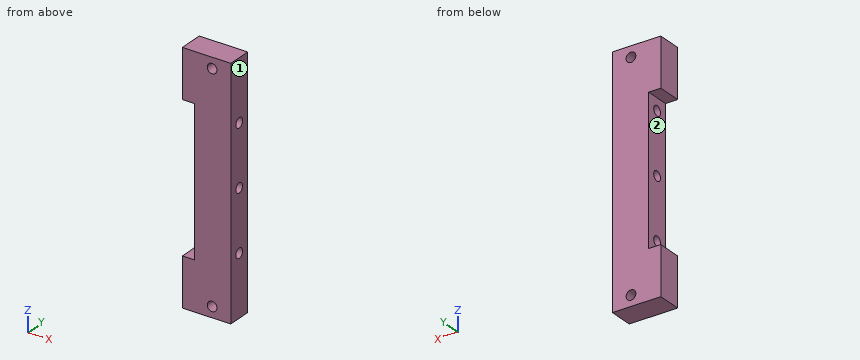
from build123d import *

# Parameters (mm, degrees)
SKETCH1_R           = 2
BOSS_EXTRUDE1_DEPTH = 10
SKETCH2_R           = 2
CUT_EXTRUDE1_DEPTH  = 30
SKETCH3_W           = 147.072515525
SKETCH3_H           = 61.375716436
CUT_EXTRUDE2_DEPTH  = 5


with BuildPart() as part:
    # Sketch1 → Boss-Extrude1 (new body)
    with BuildSketch(Plane(origin=(0, 0, 0), x_dir=(1, 0, 0), z_dir=(0, 1, 0))):
        Polygon((16.050729855, 56.814996593), (-8.949270145, 56.814996593), (-8.949270145, 36.814996593), (1.050729855, 36.814996593), (1.050729855, -23.185003407), (-8.949270145, -23.185003407), (-8.949270145, -43.185003407), (16.050729855, -43.185003407), align=None)
        with Locations((8.348885954, 52.436102934)):
            Circle(SKETCH1_R, mode=Mode.SUBTRACT)
        with Locations((8.348885954, -38.806109747)):
            Circle(SKETCH1_R, mode=Mode.SUBTRACT)
    extrude(amount=BOSS_EXTRUDE1_DEPTH)

    # Sketch2 → Cut-Extrude1 (cut)
    with BuildSketch(Plane.ZY.offset(-1.050729855)):
        with Locations((-31.814996593, 5)):
            Circle(SKETCH2_R)
        with Locations((18.185003407, 5)):
            Circle(SKETCH2_R)
        with Locations((-6.814996593, 5)):
            Circle(SKETCH2_R)
    extrude(amount=-CUT_EXTRUDE1_DEPTH, mode=Mode.SUBTRACT)

    # Sketch3 → Cut-Extrude2 (cut)
    with BuildSketch(Plane.ZY.offset(8.949270145)):
        with Locations((-8.47035824, 7.801381248)):
            Rectangle(SKETCH3_W, SKETCH3_H)
    extrude(amount=-CUT_EXTRUDE2_DEPTH, mode=Mode.SUBTRACT)


solid = part.part
Can you work these out from the model? Positions are in its coordinate system, mm. Face numbers are marked on the shaded views. Give positions to 0.01 mm unless a question says otherwise; leave off trailing zeros. Loops run counter-clockwise (first coordinate to the right, second up) from the corner with the lowest first, then second, coordinate; pieces in that order, holes last. Notation, with made-up numbers: M 27,55.5 L 74,55.5 A21 ccw 74,65.5 Z; hole C 17.5,80 d7. An arc over 180 degrees is marked long. One line per item, written item: value. Start each with the question number.
1) I'm going to push a flat-ended pin straight in: pin 1 (3 mm diameter, centred on x = 8.35, z = -52.44, fed in from -Y). Where does the tip first touch, or does it pass through?
2) If we section it at C-C, the plane x = 14.25: Write out the boundary of the cut face in (y, z) (3 decimals), and give its area (3 significant figures).
3) Thinking about a two-plate mould opening in Z: for the marked faces 1 and 2, which applies, +Z half, -Z half, draft (parallel to the pull), parting line (faces both ways), or undercut?
4) If we section it at A-A, the plane x = -1: Write out the boundary of the cut face in (y, z) (3 decimals).
5) If we section it at D-D, the plane z = -11: Write out the boundary of the cut face in (x, y), and give its area (3 significant figures).
6) If we section it at B-B, the plane y = 5: Write out the boundary of the cut face in (x, z) (3 decimals).
7) If I drill on line 1 (Z direction, x = 8.5, y = 1.75) (3 decimals); line 2 (Z direction, x = 8.5, y = 6.75) (3 decimals); line 3 (Z direction, x = 0.75, y = 7.75) (3 decimals), over which ranges is the centre line in solid material (lowest first)? Write a range as [from, to].
Completed:
1. pin 1: passes through
2. outline: M 0,-56.815 L 10,-56.815 L 10,43.185 L 0,43.185 Z; hole C 5,-31.815 d4; hole C 5,-6.815 d4; hole C 5,18.185 d4
2. area: 962 mm^2
3. face 1: draft
3. face 2: undercut
4. outline: M 0,-56.815 L 10,-56.815 L 10,-36.815 L 0,-36.815 Z; M 0,23.185 L 10,23.185 L 10,43.185 L 0,43.185 Z
5. outline: M 1.05,0 L 16.05,0 L 16.05,10 L 1.05,10 Z
5. area: 150 mm^2
6. outline: M -3.949,-56.815 L 16.051,-56.815 L 16.051,-33.815 L 1.051,-33.815 L 1.051,-36.815 L -3.949,-36.815 Z; M -3.949,23.185 L 1.051,23.185 L 1.051,20.185 L 16.051,20.185 L 16.051,43.185 L -3.949,43.185 Z; M 1.051,-29.815 L 16.051,-29.815 L 16.051,-8.815 L 1.051,-8.815 Z; M 1.051,-4.815 L 16.051,-4.815 L 16.051,16.185 L 1.051,16.185 Z; hole C 8.349,-52.436 d4; hole C 8.349,38.806 d4
7. line 1: z = [-56.815, -54.43], [-50.442, 36.812], [40.8, 43.185]
7. line 2: z = [-56.815, -54.43], [-50.442, -32.783], [-30.847, -7.783], [-5.847, 17.217], [19.153, 36.812], [40.8, 43.185]
7. line 3: z = [-56.815, -36.815], [23.185, 43.185]
